Part model, mm, in its own coordinate system. A direction names the side the tool comes from. Coordinates: 2 decimals unless noted, no trailing zeros. Order: outer loops, then holes, each group sorted by start corner. A loop starts at its lowest first (then second) coordinate and runs counter-clockwise, first axis right, second up.
1) Mould opens along X. For faces 4 (the flat face through (0, 11, 0)), 5 (the cylindrical face through (112.9, 49.656, -0.044)), 6 (the flat face through (6.35, 15, -9)) say: +X half, -X half, draft (parallel to the pull), parting line (faces both ways), or undercut.
2) Cut at A-A (z = 12.7). List the corners of the cut face in (x, y) (3 decimals), and give its area (3 significant figures).
3) Cut at C-C (y = 21). List the corners of the cut face in (x, z) (3 decimals), and give its area (3 significant figures).
4) Tool access for faces 1 (the conical face through (4.583, 14.057, -11.22)), 2 (the flat face through (62, 32, -3.175)), 3 (the flat face through (6.35, 10, 9)): list every direction of +Z, -Z, +X, -X, +Y, -Y with a clear straight run to the whole face (end or side of a thin tool).
5) Cut at D-D (x = 70.5). List the corners of the cut face in (y, z) (3 decimals).
6) Cut at B-B (y = 12.7). List the corners of the cut face in (x, z) (3 decimals), and give its area (3 significant figures).
7) Wall check: L1, parallel to Z at x = 1.6, y = 12.7 (3 decimals); L2, parallel to Z at x = 1, y = 12; L3, parallel to X at y = 15, z = 8.5. Give the ranges that are in metal, low to high.
8) Pin check, flat tips, straight feed: pin 1 Ø8 at (y, z) = (17.5, -11.5) entering from +X; pin 2 Ø5 at (x, z) = (54.5, -4.5) entering from -Y; pin 3 Ø2 at (x, z) = (87, 3.5) entering from +Y. Stop position of each tip, or through.
Autodesk Inventor part; units mm, degrees
ref_plane "YZ Plane" through (0, 0, 0) normal (1, 0, 0) x (0, 1, 0)
ref_plane "XZ Plane" through (0, 0, 0) normal (0, 1, 0) x (-1, 0, 0)
ref_plane "XY Plane" through (0, 0, 0) normal (0, 0, 1) x (1, 0, 0)
sketch "Sketch5" plane through (0, 0, 0) normal (0, 0, 1) x (1, 0, 0)
  line L0 (0, 0) -> (6.35, 0)
  line L1 (6.35, 0) -> (6.35, 25.4)
  line L2 (6.35, 25.4) -> (0, 25.4)
  line L3 (0, 25.4) -> (0, 0)
  dimension "d21" = 25.4
  dimension "d22" = 6.35
extrude "Extrusion3" add sketch "Sketch5" against normal mid plane 38.1
sketch "Sketch6" plane through (0, 0, 0) normal (0, 0, 1) x (1, 0, 0)
  line L0 (6.35, 25.4) -> (6.35, 0)
  line L1 (0, 25.4) -> (6.35, 25.4)
  line L2 (6.35, 0) -> (0, 0)
  line L3 (0, 0) -> (0, 25.4)
  line L4 (6.35, 0) -> (127.9525, 44.2597)
  line L5 (6.35, 0) -> (135.7567, 0) construction
  line L6 (127.9525, 69.6597) -> (127.9525, 44.2597)
  arc A0 (95.1208, 57.7099) -> (120.7792, 67.0488) centre (107.95, 62.3794) ccw
  line L7 (6.35, 25.4) -> (95.1208, 57.7099)
  line L8 (120.7792, 67.0488) -> (127.9525, 69.6597)
  dimension "d25" = 20
  dimension "d26" = 27.305
  dimension "d29" = 6.35
  dimension "d30" = 107.95
  dimension "d33" = 0
extrude "Extrusion4" add sketch "Sketch6" along normal mid plane 6.35 contours L7 A0 L8 L6 L4 L0
sketch "Sketch7" plane through (6.35, 0, 19.05) normal (1, 0, 0) x (0, 0, -1)
  line L0 (38.1, 25.4) -> (0, 25.4) construction
  line L1 (6.35, 25.4) -> (6.35, 0) construction
  line L2 (31.75, 25.4) -> (31.75, 0) construction
  line L3 (0, 0) -> (0, 25.4) construction
  line L4 (38.1, 25.4) -> (38.1, 0) construction
  line L5 (0, 0) -> (15.875, 0)
  line L6 (22.225, 0) -> (38.1, 0)
  point P0 (19.05, 0)
  point P1 (6.35, 12.7)
  point P2 (31.75, 12.7)
  dimension "d34" = 6.35
  dimension "d35" = 6.35
sketch "Sketch8" plane through (0, 0, 0) normal (0, 0, 1) x (1, 0, 0)
  line L0 (0, 0) -> (0, 25.4)
  line L1 (6.35, 0) -> (0, 0)
  line L2 (127.9525, 44.2597) -> (6.35, 0)
  line L3 (0, 0) -> (6.35, 0)
  line L4 (0, -2.3112) -> (6.35, 0)
  line L5 (0, 0) -> (0, -2.3112)
extrude "Extrusion5" add sketch "Sketch8" along normal mid plane 38.1
hole "Hole3" at (6.35, 12.7, 12.7) at (6.35, 12.7, -12.7) direction (-1, 0, 0) diameter 3.81 end through all countersink diameter 7.0866 countersink angle 82
sketch "Sketch9" plane through (0, 0, 0) normal (0, 0, 1) x (1, 0, 0)
  line L0 (6.35, 25.4) -> (6.35, 0)
  line L1 (0, 25.4) -> (6.35, 25.4)
  line L2 (6.35, 25.4) -> (95.1208, 57.7099)
  line L3 (0, -2.3112) -> (0, 25.4)
  line L4 (6.35, 25.4) -> (0, 25.4)
  line L5 (6.35, 25.4) -> (6.35, 0)
  line L6 (6.35, 25.4) -> (0, 23.0888)
  line L7 (0, 25.4) -> (0, 23.0888)
  point P0 (0, 0)
extrude "Extrusion6" cut sketch "Sketch9" along normal mid plane 38.1
equation "\"d21\" = supportHeight"
equation "\"d22\" = supportWidth"
equation "\"d23\" = totalScrewHoldWidth"
equation "\"d25\" = supportAngle"
equation "\"d26\" = pipeDiameter"
equation "\"d30\" = distanceFromWallToPipeCenter"
equation "\"d31\" = supportWidth"
equation "\"d47\" = totalScrewHoldWidth"
equation "\"d63\" = totalScrewHoldWidth"
equation "\"pipeDiameter\" = 27.305"
equation "\"distanceFromWallToPipeCenter\" = 107.95"
equation "\"supportHeight\" = 25.4"
equation "\"supportWidth\" = 6.35"
equation "\"screwHoldDepth\" = 6.35"
equation "\"totalScrewHoldWidth\" = 38.1"
equation "\"screwPositionFromTop\" = 6.35"
equation "\"supportAngle\" = 20deg"
properties part number "PipeSupport-4_00-020"
Geometry check:
1. face 4: -X half
1. face 5: undercut
1. face 6: +X half
2. outline: (0, -2.311) - (6.35, 0) - (6.35, 9.157) - (4.465, 10.795) - (0, 10.795) - close; (0, 14.605) - (4.465, 14.605) - (6.35, 16.243) - (6.35, 25.4) - (0, 23.089) - close
2. area: 134 mm2
3. outline: (0, -19.05) - (6.35, -19.05) - (6.35, -3.175) - (64.047, -3.175) - (64.047, 3.175) - (6.35, 3.175) - (6.35, 19.05) - (0, 19.05) - close
3. area: 608 mm2
4. face 1: +X
4. face 2: -Z, +X, +Y, -Y
4. face 3: +Z, +X, +Y, -Y
5. outline: (23.349, -3.175) - (48.749, -3.175) - (48.749, 3.175) - (23.349, 3.175) - close
6. outline: (0, -19.05) - (6.35, -19.05) - (6.35, -16.243) - (4.465, -14.605) - (0, -14.605) - close; (0, -10.795) - (4.465, -10.795) - (6.35, -9.157) - (6.35, -3.175) - (41.243, -3.175) - (41.243, 3.175) - (6.35, 3.175) - (6.35, 9.157) - (4.465, 10.795) - (0, 10.795) - close; (0, 14.605) - (4.465, 14.605) - (6.35, 16.243) - (6.35, 19.05) - (0, 19.05) - close
6. area: 409 mm2
7. L1: z = -19.05 to -14.605, -10.795 to 10.795, 14.605 to 19.05
7. L2: z = -19.05 to -14.47, -10.93 to 10.93, 14.47 to 19.05
7. L3: x = 0 to 6.35
8. pin 1: stops at x = 6.35
8. pin 2: stops at y = 16.75
8. pin 3: stops at y = 55.1
